from build123d import *

# Parameters (mm, degrees)
SKETCH1_W                = 19.05
SKETCH1_H                = 19.05
SKETCH1_W_2              = 15.875
SKETCH1_H_2              = 15.875
BOSS_EXTRUDE1_DEPTH      = 66.7766
SKETCH2_R                = 2.8956
BASEPLATEMOUNTHOLE_DEPTH = 20.05
CUT_EXTRUDE1_REACH       = 21.05
SKETCH3_R                = 4.7625


with BuildPart() as part:
    # Sketch1 → Boss-Extrude1 (new body, symmetric)
    with BuildSketch(Plane(origin=(0, 0, 0), x_dir=(0, -1, 0), z_dir=(0, 0, 1))):
        Rectangle(SKETCH1_W, SKETCH1_H)
        Rectangle(SKETCH1_W_2, SKETCH1_H_2, mode=Mode.SUBTRACT)
    extrude(amount=BOSS_EXTRUDE1_DEPTH, both=True)

    # Sketch2 → BasePlateMountHole (cut, through all)
    with BuildSketch(Plane(origin=(0, 9.525, 0), x_dir=(1, 0, 0), z_dir=(0, 1, 0))):
        with Locations((0, -34.8234)):
            Circle(SKETCH2_R)
    extrude(amount=-BASEPLATEMOUNTHOLE_DEPTH, mode=Mode.SUBTRACT)

    # Sketch3 → Cut-Extrude1 (cut, up to next)
    with BuildSketch(Plane.ZY.offset(9.525), mode=Mode.PRIVATE) as cut_extrude1_sk1:
        with Locations((3.3782, 0)):
            Circle(SKETCH3_R)
    cut_extrude1_tool1 = extrude(cut_extrude1_sk1.sketch, amount=-CUT_EXTRUDE1_REACH, mode=Mode.PRIVATE) & part.part
    add(cut_extrude1_tool1.solids().sort_by_distance((-9.525, 0, 3.3782))[0], mode=Mode.SUBTRACT)


solid = part.part
Work out the finished part from the listing and answer in its coordinate system (mm). A direction names the side the tool comes from. Give positions to 0.01 mm unless a question says otherwise; leave off trailing zeros. Loops run counter-clockwise (first coordinate to the right, second up) from the corner with the lowest first, then second, coordinate; pieces in that order, holes last. Notation, with made-up numbers: (-34, 64) -> (-21, 64) arc R20 cw to (-21, 79) -> close; hole circle Ø10 at (-39.75, -10). An arc over 180 degrees is marked (long way). Use a Markdown table: item, result. Add a question column.
1. For faces 1 (the flat face through (0, 9, -66.777)), 2 (the flat face through (7.938, 0, 1)), 3 (the cylindrical face through (-8.7, -2.9, -0.4)), determine the directions among +Z, -Z, +X, -X, +Y, -Y from which every point of the face is accessible in a straight line to the end or side of a thin tool.
2. Section D-D on x = 0 is taken. Determine the outline of the cut face in (y, z) (1 decimal), and give its area (3 significant figures).
3. Section A-A on y = 0 is taken. Determine the outline of the cut face in (x, z) (1 decimal).
4. Section B-B on x = 6 is taken. Determine the outline of the cut face in (y, z) (1 decimal).
5. Find the intervals of material crossed by probe 1 along X at (y, z) = (-6.5, 10) (1 decimal); probe 2 along Z at (x, y) = (0, -8.7), in increasing order.
6. Determine the mould class of faces 4 (the flat face through (-7.938, -5, 1)), 5 (the flat face through (9.525, 0, 1)), 6 (the flat face through (0, 9, 66.777)) for opening direction X: released by +X, released by -X, zero draft, split by the parting line, or undercut.
7. A flat-ended cylindrical pin translates along its axis: pin 1 Ø4.5 at (x, z) = (0, 34.82) entering from +Y. Find the tip coordinate at first contact, or state that the pin passes through.
8. Section C-C on z = -35.5 is taken. Determine the outline of the cut face in (x, y) (1 decimal), and give its area (3 significant figures).
Results below:
| question | item | result |
|---|---|---|
| 1 | face 1 | -Z, +X, -X, +Y, -Y |
| 1 | face 2 | +Z, -Z |
| 1 | face 3 | -X |
| 2 | outline | (-9.5, -66.8) -> (-7.9, -66.8) -> (-7.9, 31.9) -> (-9.5, 31.9) -> close; (-9.5, 37.7) -> (-7.9, 37.7) -> (-7.9, 66.8) -> (-9.5, 66.8) -> close; (7.9, -66.8) -> (9.5, -66.8) -> (9.5, 31.9) -> (7.9, 31.9) -> close; (7.9, 37.7) -> (9.5, 37.7) -> (9.5, 66.8) -> (7.9, 66.8) -> close |
| 2 | area | 406 mm^2 |
| 3 | outline | (-9.5, -66.8) -> (-7.9, -66.8) -> (-7.9, -1.4) -> (-9.5, -1.4) -> close; (-9.5, 8.1) -> (-7.9, 8.1) -> (-7.9, 66.8) -> (-9.5, 66.8) -> close; (7.9, -66.8) -> (9.5, -66.8) -> (9.5, 66.8) -> (7.9, 66.8) -> close |
| 4 | outline | (-9.5, -66.8) -> (-7.9, -66.8) -> (-7.9, 66.8) -> (-9.5, 66.8) -> close; (7.9, -66.8) -> (9.5, -66.8) -> (9.5, 66.8) -> (7.9, 66.8) -> close |
| 5 | probe 1 | x = -9.5 to -7.9, 7.9 to 9.5 |
| 5 | probe 2 | z = -66.78 to 31.93, 37.72 to 66.78 |
| 6 | face 4 | undercut |
| 6 | face 5 | released by +X |
| 6 | face 6 | zero draft |
| 7 | pin 1 | passes through |
| 8 | outline | (-9.5, -9.5) -> (9.5, -9.5) -> (9.5, 9.5) -> (-9.5, 9.5) -> close; hole (-7.9, -7.9) -> (7.9, -7.9) -> (7.9, 7.9) -> (-7.9, 7.9) -> close |
| 8 | area | 111 mm^2 |
